```python
from build123d import *

# Parameters (mm, degrees)
SKETCH_1_W      = 20
SKETCH_1_H      = 15
EXTRUDE_1_DEPTH = 3
CHAMFER_1_SIZE  = 3


with BuildPart() as part:
    # 草图1 → 凸台-拉伸1 (new, symmetric)
    with BuildSketch(Plane.XY):
        Rectangle(SKETCH_1_W, SKETCH_1_H)
    extrude(amount=EXTRUDE_1_DEPTH, both=True)

    # 倒角1
    chamfer_1_edges = [part.edges().sort_by_distance(p)[0] for p in [
        (10, 7.5, 0),
    ]]
    chamfer(chamfer_1_edges, length=CHAMFER_1_SIZE)


solid = part.part
```
Here's how the part is built. I have some questions about the finished solid (model axes, mm). Round coordinates to 2 decimals unless told otherwise and drop trailing zeros. Write each loop counter-clockwise with the first axis right and the second up, starting at its lowest first coordinate (ties: lowest second). Pieces come first, ordered by that corner, then holes. Notation, with made-up numbers: M 48.5,-38 L 100.5,-38 A30 ccw 100.5,-7 Z; hole C -18.75,-0.75 d1. An arc over 180 degrees is marked long. Answer as CSV lines item,"result". Start each with the question number.
1. Suppose I cut it at A-A on z = -0.4. Write out the boundary of the cut face in (x, y), then the cut area to 4 significant figures.
2. I need wall thicknesses on probe 1 along Y at (x, z) = (7.5, -1.6); probe 2 along Y at (x, z) = (8.5, -1.25); probe 3 along X at (y, z) = (6.75, -1.5). Which ranges of each line are inside material? Lowest first, please.
3. Suppose I cut it at B-B on y = 5. Write out the boundary of the cut face in (x, z).
Check result:
1,outline,"M -10,-7.5 L 10,-7.5 L 10,4.5 L 7,7.5 L -10,7.5 Z"
1,area,"295.5 mm2"
2,probe 1,"y = -7.5 to 7"
2,probe 2,"y = -7.5 to 6"
2,probe 3,"x = -10 to 7.75"
3,outline,"M -10,-3 L 9.5,-3 L 9.5,3 L -10,3 Z"
